Source: CAD feature listing. Evaluate the final solid. Frame: model axes, mm. A direction names the side the tool comes from. Give positions to 0.01 mm unless a question says otherwise; leave off trailing zeros.
1) First-contact query: P1, Ø1.5, axis at x = -15, z = -0.5, coming from the +Y side; P2, Ø3, axis at x = -36, y = 3.5, coming from the -Z side; P3, Ø0.7, axis at x = 49, y = 6, coming from the -Z side. Flat tips, straight axial feed; report the tip coordinate or a pass-through.
2) Material intervals for line 1 (X direction, y = 4.25, z = -1.5); line 2 (Y direction, x = 16.5, z = -0.5); line 3 (Z direction, x = -26.5, y = 5.5), sorted ascending.
3) Draft query along Z for faces 1 (the face through (-30.5, 5.6, 0.1)), 2 (the face through (32.007, 3.562, -5.586)), 3 (the face through (68, 0, 0)). Return one class per face: released by +Z, released by -Z, zero draft, split by the parting line, or undercut.
4) Access query for faces 4 (the face through (18, 4.2, 0)), 5 (the face through (0.441, -6.834, 1.517)), 6 (the face through (-31.993, 3.562, -5.586)). Directions: +Z, -Z, +X, -X, +Y, -Y. A direction counts if a zero-diameter tool reaches every point of the face in a straight line with its end or side. Return the directions, or none.
```python
from build123d import *

# Parameters (mm, degrees)
SKETCH1_R           = 7
BOSS_EXTRUDE1_DEPTH = 34
CUT_EXTRUDE1_DEPTH  = 2.8
SKETCH5_R           = 7
BOSS_EXTRUDE3_DEPTH = 20
SKETCH7_R           = 7
BOSS_EXTRUDE4_DEPTH = 34
SKETCH11_W          = 1
SKETCH11_H          = 0.75
CHAMFER1_SIZE       = 1
CUT_EXTRUDE3_DEPTH  = 2.8


with BuildPart() as part:
    # Sketch1 → Boss-Extrude1 (new body, symmetric)
    with BuildSketch(Plane(origin=(0, 0, 0), x_dir=(0, 0, -1), z_dir=(1, 0, 0))):
        Circle(SKETCH1_R)
    extrude(amount=BOSS_EXTRUDE1_DEPTH, both=True)

    # Sketch4 → Cut-Extrude1 (cut)
    with BuildSketch(Plane(origin=(0, 7, 0), x_dir=(1, 0, 0), z_dir=(0, 1, 0))):
        with BuildLine():
            Line((-28, 2.5), (-8, 2.5))
            ThreePointArc((-8, 2.5), (-5.5, 0), (-8, -2.5))
            Line((-8, -2.5), (-28, -2.5))
            ThreePointArc((-28, -2.5), (-30.5, 0), (-28, 2.5))
        make_face()
    cut_extrude1 = extrude(amount=-CUT_EXTRUDE1_DEPTH, mode=Mode.SUBTRACT)

    # Mirror1: Cut-Extrude1 across plane
    add(cut_extrude1.mirror(Plane(origin=(0, 0, 0), x_dir=(0, 0, 1), z_dir=(1, 0, 0))), mode=Mode.SUBTRACT)

    # Sketch5 → Boss-Extrude3 (add)
    with BuildSketch(Plane.ZY.offset(34)):
        Circle(SKETCH5_R)
    extrude(amount=BOSS_EXTRUDE3_DEPTH)

    # Sketch7 → Boss-Extrude4 (add)
    with BuildSketch(Plane(origin=(34, 0, 0), x_dir=(0, 0, -1), z_dir=(1, 0, 0))):
        Circle(SKETCH7_R)
    extrude(amount=BOSS_EXTRUDE4_DEPTH)

    # Sketch11 → Cut-Revolve1 (revolve, cut)
    with BuildSketch(Plane.XY):
        with Locations((63, 7)):
            Rectangle(SKETCH11_W, SKETCH11_H)
        with Locations((32, 7)):
            Rectangle(SKETCH11_W, SKETCH11_H)
        with Locations((-32, 7)):
            Rectangle(SKETCH11_W, SKETCH11_H)
    revolve(axis=Axis((71.5, 0, 0), (-1, 0, 0)), mode=Mode.SUBTRACT)

    # Chamfer1
    chamfer1_edges = [part.edges().sort_by_distance(p)[0] for p in [
        (-54, 0, -7),
        (68, 0, 7),
    ]]
    chamfer(chamfer1_edges, length=CHAMFER1_SIZE)

    # Sketch9 → Cut-Extrude3 (cut)
    with BuildSketch(Plane(origin=(0, 7, 0), x_dir=(1, 0, 0), z_dir=(0, 1, 0))):
        with BuildLine():
            Line((37.5, 2.5), (57.5, 2.5))
            ThreePointArc((57.5, 2.5), (60, 0), (57.5, -2.5))
            Line((57.5, -2.5), (37.5, -2.5))
            ThreePointArc((37.5, -2.5), (35, 0), (37.5, 2.5))
        make_face()
    extrude(amount=-CUT_EXTRUDE3_DEPTH, mode=Mode.SUBTRACT)


solid = part.part
```
From the geometry:
1. P1: stops at y = 4.2
1. P2: stops at z = -6.71
1. P3: stops at z = -4.13
2. line 1: x = -54 to -30, -6 to 6, 30 to 35.5, 59.5 to 68
2. line 2: y = -6.98 to 4.2
2. line 3: z = -4.33 to -2.5, 2.5 to 4.33
3. face 1: undercut
3. face 2: split by the parting line
3. face 3: zero draft
4. face 4: +Y
4. face 5: +X, -X
4. face 6: none
